The model under review builds one solid part; all positions refer to its coordinate system, in mm. A direction names the side the tool comes from. Give positions to 0.01 mm unless a question says otherwise; leave off trailing zeros. Loops run counter-clockwise (first coordinate to the right, second up) from the corner with the lowest first, then second, coordinate; pieces in that order, holes last. Notation, with made-up numbers: M 57,17 L 97,17 A13 ccw 97,42 Z; hole C 7.25,-8 d7. An arc over 180 degrees is marked long. One line per item, written item: value. Start each with the question number.
Q1. We need section A-A on y = 0. Give the number of separate pieces and of enclosed holes in the cut face, plus the area to 3 significant figures.
Q2. To check wall thickness, follow line 1 along Y through (x, z) = (-13.5, 43); line 2 along X through (y, z) = (0, 106.5); line 3 along X through (y, z) = (0, 91) (3 decimals). State the ranges of each line that lie inside material, in increasing order. Write a range as from..to.
Q3. We need section B-B on x = 0. Write out the cut boundary in (y, z) (3 decimals), plus the area to 3 significant figures.
Q4. Mouldability with a two-part tool opening along X and no side actions: class faces 3 (the face through (2.5, -14, 75)), 4 (the face through (12, 5, 75)), 5 (the face through (15, 9, 75)), 6 (the face through (-4.07, -0.03, 66.18)) as released by +X, released by -X, zero draft, split by the parting line, or undercut.
Q5. We need section D-D on y = -6.5. Write out the cut boundary in (x, z).
Q6. We need section C-C on x = 12.75. Write out the cut boundary in (y, z), plus the area to 4 significant figures.
Q7. For pin 1 (3.5 mm diameter, centred on y = 0, z = 75.04, fed in from +X), flat-tipped, find the tip position at first contact; note if it passes through.
Q8. For faces 1 (the face through (-9, -15, 75)), 2 (the face through (8.09, 5.26, 74.52)), list the 3-axis set-ups (+Z, -Z, +X, -X, +Y, -Y) from which the entire face can be reached by the end or side of a thin tool; tool diameter is ignored.
```python
from build123d import *

# Parameters (mm, degrees)
BOSS_EXTRUDE1_DEPTH = 150
SKETCH2_R           = 3.75
CUT_EXTRUDE1_DEPTH  = 151
SKETCH3_R           = 4
CUT_EXTRUDE2_DEPTH  = 61
SKETCH5_R           = 4
CUT_EXTRUDE5_DEPTH  = 20
SKETCH6_R           = 4
CUT_EXTRUDE6_DEPTH  = 20
SCALE1_SCALE        = 0.5


with BuildPart() as part:
    # Sketch1 → Boss-Extrude1 (new body)
    with BuildSketch(Plane.XY):
        with BuildLine():
            Line((-5, 30), (-5, 24))
            Line((-5, 24), (-15.928932188, 24))
            ThreePointArc((-15.928932188, 24), (-16.852811721, 23.382683432), (-16.636038969, 22.292893219))
            Line((-16.636038969, 22.292893219), (-4.242640687, 9.899494937))
            ThreePointArc((-4.242640687, 9.899494937), (0, 8.142135624), (4.242640687, 9.899494937))
            Line((4.242640687, 9.899494937), (16.636038969, 22.292893219))
            ThreePointArc((16.636038969, 22.292893219), (16.852811721, 23.382683432), (15.928932188, 24))
            Line((15.928932188, 24), (5, 24))
            Line((5, 24), (5, 30))
            Line((5, 30), (30, 30))
            Line((30, 30), (30, 5))
            Line((30, 5), (24, 5))
            Line((24, 5), (24, 15.928932188))
            ThreePointArc((24, 15.928932188), (23.382683432, 16.852811721), (22.292893219, 16.636038969))
            Line((22.292893219, 16.636038969), (9.899494937, 4.242640687))
            ThreePointArc((9.899494937, 4.242640687), (8.142135624, 0), (9.899494937, -4.242640687))
            Line((9.899494937, -4.242640687), (22.292893219, -16.636038969))
            ThreePointArc((22.292893219, -16.636038969), (23.382683432, -16.852811721), (24, -15.928932188))
            Line((24, -15.928932188), (24, -5))
            Line((24, -5), (30, -5))
            Line((30, -5), (30, -30))
            Line((30, -30), (5, -30))
            Line((5, -30), (5, -24))
            Line((5, -24), (15.928932188, -24))
            ThreePointArc((15.928932188, -24), (16.852811721, -23.382683432), (16.636038969, -22.292893219))
            Line((16.636038969, -22.292893219), (4.242640687, -9.899494937))
            ThreePointArc((4.242640687, -9.899494937), (0, -8.142135624), (-4.242640687, -9.899494937))
            Line((-4.242640687, -9.899494937), (-16.636038969, -22.292893219))
            ThreePointArc((-16.636038969, -22.292893219), (-16.852811721, -23.382683432), (-15.928932188, -24))
            Line((-15.928932188, -24), (-5, -24))
            Line((-5, -24), (-5, -30))
            Line((-5, -30), (-30, -30))
            Line((-30, -30), (-30, -5))
            Line((-30, -5), (-24, -5))
            Line((-24, -5), (-24, -15.928932188))
            ThreePointArc((-24, -15.928932188), (-23.382683432, -16.852811721), (-22.292893219, -16.636038969))
            Line((-22.292893219, -16.636038969), (-9.899494937, -4.242640687))
            ThreePointArc((-9.899494937, -4.242640687), (-8.142135624, 0), (-9.899494937, 4.242640687))
            Line((-9.899494937, 4.242640687), (-22.292893219, 16.636038969))
            ThreePointArc((-22.292893219, 16.636038969), (-23.382683432, 16.852811721), (-24, 15.928932188))
            Line((-24, 15.928932188), (-24, 5))
            Line((-24, 5), (-30, 5))
            Line((-30, 5), (-30, 30))
            Line((-30, 30), (-5, 30))
        make_face()
    extrude(amount=BOSS_EXTRUDE1_DEPTH)

    # Sketch2 → Cut-Extrude1 (cut, through all)
    with BuildSketch(Plane(origin=(0, 0, 0), x_dir=(-1, 0, 0), z_dir=(0, 0, -1))):
        Circle(SKETCH2_R)
    extrude(amount=-CUT_EXTRUDE1_DEPTH, mode=Mode.SUBTRACT)

    # Sketch3 → Cut-Extrude2 (cut, through all)
    with BuildSketch(Plane.ZY.offset(30)):
        with Locations(Location((75, 0, 0), (0, 0, 270))):  # turned: the seam where the file's is
            Circle(SKETCH3_R)
        with Locations(Location((30, 0, 0), (0, 0, 270))):  # turned: the seam where the file's is
            Circle(SKETCH3_R)
    extrude(amount=-CUT_EXTRUDE2_DEPTH, mode=Mode.SUBTRACT)

    # Sketch5 → Cut-Extrude5 (cut)
    with BuildSketch(Plane(origin=(0, 0, 0), x_dir=(-1, 0, 0), z_dir=(0, 0, -1))):
        Circle(SKETCH5_R)
    extrude(amount=-CUT_EXTRUDE5_DEPTH, mode=Mode.SUBTRACT)

    # Sketch6 → Cut-Extrude6 (cut)
    with BuildSketch(Plane.XY.offset(150)):
        with Locations(Location((0, 0, 0), (0, 0, 180))):  # turned: the seam where the file's is
            Circle(SKETCH6_R)
    extrude(amount=-CUT_EXTRUDE6_DEPTH, mode=Mode.SUBTRACT)


with BuildPart() as part_1:
    # Scale1: scaled about (5.21e-07, -1.92e-07, 75.081821445)
    add(part.part.scale(SCALE1_SCALE).moved(Location((2.6e-07, -9.6e-08, 37.540910723))))


solid = part_1.part
```
Solved:
1. separate pieces: 6
1. enclosed holes: 0
1. area: 289 mm2
2. line 1: -15..-2.5, 2.5..15
2. line 2: -4.07..-2, 2..4.07
2. line 3: -4.071..-1.875, 1.875..4.071
3. outline: M -4.071,37.541 L -2,37.541 L -2,47.541 L -1.875,47.541 L -1.875,51.845 A2 cw -1.875,53.237 L -1.875,74.345 A2 cw -1.875,75.737 L -1.875,102.541 L -2,102.541 L -2,112.541 L -4.071,112.541 Z; M 1.875,47.541 L 2,47.541 L 2,37.541 L 4.071,37.541 L 4.071,112.541 L 2,112.541 L 2,102.541 L 1.875,102.541 L 1.875,75.737 A2 cw 1.875,74.345 L 1.875,53.237 A2 cw 1.875,51.845 Z
3. area: 324 mm2
4. face 3: undercut
4. face 4: undercut
4. face 5: released by +X
4. face 6: released by -X
5. outline: M -15,37.54 L -12,37.54 L -12,112.54 L -15,112.54 Z; M -9.33,37.54 L -3.67,37.54 L -3.67,112.54 L -9.33,112.54 Z; M 3.67,37.54 L 9.33,37.54 L 9.33,112.54 L 3.67,112.54 Z; M 12,37.54 L 15,37.54 L 15,112.54 L 12,112.54 Z
6. outline: M -15,37.54 L -2.5,37.54 L -2.5,112.54 L -15,112.54 Z; M 2.5,37.54 L 15,37.54 L 15,112.54 L 2.5,112.54 Z
6. area: 1,875 mm2
7. pin 1: through
8. face 1: +Z, -Z, +X, -X, -Y
8. face 2: +Z, -Z
